For this review, take the finished solid that the model builds, in its own axes (mm). Face numbers are marked on the shaded views. Round coordinates to 2 decimals unless told otherwise and drop trailing zeros. Write each loop counter-clockwise with the first axis right and the second up, starting at its lowest first coordinate (ties: lowest second). Pieces come first, ordered by that corner, then holes. Notation, with made-up numbers: (50, 25) -> (86, 25) arc R21 ccw to (86, 48) -> close; hole circle Ø11 at (12, -39.5). An arc over 180 degrees is marked (long way). Answer as CSV lines item,"result". Start each with the question number.
Item 1: Wall thickness on probe 1 along Z at (x, y) = (0, 1.4); probe 2 along Z at (x, y) = (-0.5, 1); probe 3 along X at (y, z) = (0.2, 0.5): over which ranges is each line inside the solid? List them lowest first. Write a range as from..to.
Item 2: Take a section at A-A on x = 0.75. Give the boundary of the cut face in (y, z), then the cut area to 3 significant figures.
Item 3: Take a section at D-D on x = 3. Give the boundary of the cut face in (y, z).
Item 4: Take a section at B-B on y = 1.45. Give the boundary of the cut face in (x, z).
Item 5: For pin 1 Ø1 at (y, z) = (1, 0) entering from -X, flat-tipped, find the tip position at first contact; note if it passes through.
Item 6: Mouldability with a two-part tool opening along Z and no side actions: class the marked faces 1, 2 and 3 as +Z half, -Z half, draft (parallel to the pull), parting line (faces both ways), or undercut.
Item 7: Take a section at C-C on z = 1.5. Give the boundary of the cut face in (x, y).
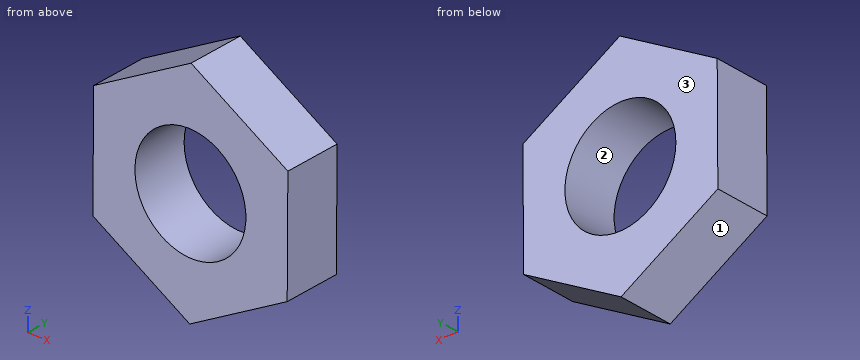
Autodesk Inventor part; units mm, degrees
ref_plane "YZ Plane" through (0, 0, 0) normal (1, 0, 0) x (0, 1, 0)
ref_plane "XZ Plane" through (0, 0, 0) normal (0, 1, 0) x (-1, 0, 0)
ref_plane "XY Plane" through (0, 0, 0) normal (0, 0, 1) x (1, 0, 0)
sketch "Sketch1" plane through (0, 0, 0) normal (0, 1, 0) x (-1, 0, 0)
  circle A0 centre (0, 0) radius 2
  line L0 (3.5123, -2) -> (0.0241, -4.0418)
  line L1 (0.0241, -4.0418) -> (-3.4882, -2.0418)
  line L2 (-3.4882, -2.0418) -> (-3.5123, 2)
  line L3 (-3.5123, 2) -> (-0.0241, 4.0418)
  line L4 (-0.0241, 4.0418) -> (3.4882, 2.0418)
  line L5 (3.4882, 2.0418) -> (3.5123, -2)
  dimension "d0" = 4
extrude "Extrusion1" add sketch "Sketch1" along normal blind 2
properties part number "hex"
Output values:
1,probe 1,"z = -4.03..-2, 2..4.03"
1,probe 2,"z = -3.76..-1.94, 1.94..3.74"
1,probe 3,"x = -3.5..-1.94, 1.94..3.5"
2,outline,"(0, -3.6) -> (2, -3.6) -> (2, -1.85) -> (0, -1.85) -> close; (0, 1.85) -> (2, 1.85) -> (2, 3.62) -> (0, 3.62) -> close"
2,area,"7.02 mm^2"
3,outline,"(0, -2.32) -> (2, -2.32) -> (2, 2.3) -> (0, 2.3) -> close"
4,outline,"(-3.51, -2) -> (-0.02, -4.04) -> (3.49, -2.04) -> (3.51, 2) -> (0.02, 4.04) -> (-3.49, 2.04) -> close; hole circle Ø4 at (0, 0)"
5,pin 1,"stops at x = -3.5"
6,face 1,"-Z half"
6,face 2,"undercut"
6,face 3,"draft"
7,outline,"(-3.49, 0) -> (-1.32, 0) -> (-1.32, 2) -> (-3.49, 2) -> close; (1.32, 0) -> (3.51, 0) -> (3.51, 2) -> (1.32, 2) -> close"
